Check sheet for the modelled part. Datum: model origin and axes. Units: mm. Face numbers are marked on the shaded views. Round coordinates to 2 decimals unless told otherwise and drop trailing zeros. Order: outer loops, then holes, each group sorted by start corner. A loop starts at its lowest first (then second) coordinate and runs counter-clockwise, first axis right, second up. Notation, with made-up numbers: M -7,-12.5 L 36,-12.5 A16 ccw 36,4.5 Z; hole C 28,73.5 d1. An arc over 180 degrees is marked long. One line per item, written item: value. Start each with the question number.
(1) Cross-section at B-B, the plane x = 65. Enter the section's corners in (y, z), and give its area (3 significant figures).
(2) Depth check by flat-ended pin: pin 1 Ø23.5 at (x, y) = (-6.5, 0) entering from +Z; pin 2 Ø4.5 at (y, z) = (-13.5, 4) entering from +X; pin 3 Ø2 at (x, z) = (-23, 6) entering from -Y. Enter the tip coordinate at first touch or a pass-through.
(3) Cross-section at A-A, the plane x = 15.5. Enter the section's corners in (y, z).
(4) Thickness scan on L1, parallel to X at y = -8, z = 3.75; L2, parallel to Z at x = 9, y = -16.5. Record the ranges inside material, lowest first.
(5) Release check for a two-part mould opening along X. For the marked faces 1 and 2 record: released by +X, released by -X, zero draft, split by the parting line, or undercut.
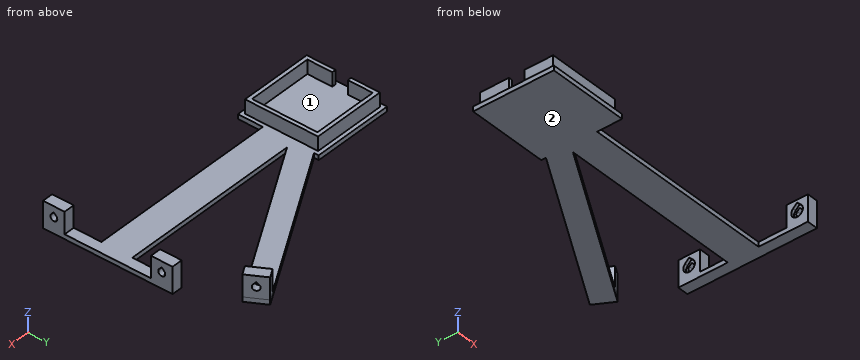
from build123d import *

# Parameters (mm, degrees)
F1_DEPTH  = 9
F2_W      = 123.8
F2_H      = 10
F3_DEPTH  = 3
F5_DEPTH  = 5
F6_W      = 14
F6_H      = 14
F7_DEPTH  = 2
F10_DEPTH = 2
F11_W     = 14
F11_H     = 14
F12_DEPTH = 5


with BuildPart() as f1:
    # F0 (on Top) → F1 (new body)
    with BuildSketch(Plane.XY):
        Polygon((-21.2, 21.2), (21.2, 21.2), (21.2, 0), (23.7, 0), (23.7, 23.7), (-23.7, 23.7), (-23.7, 5), (-21.2, 5), align=None)
        Polygon((23.7, 0), (21.2, 0), (21.2, -21.2), (-21.2, -21.2), (-21.2, -5), (-23.7, -5), (-23.7, -23.7), (23.7, -23.7), align=None)
    extrude(amount=F1_DEPTH)

    # F2 (on Top) → F3 (join)
    with BuildSketch(Plane.XY):
        Polygon((-26.2, 26.2), (-26.2, -26.2), (26.2, -26.2), (26.2, -10), (26.2, 0), (0, 0), (26.2, 15.1265770528), (26.2, 23.2094808214), (26.2, 26.2), align=None)
        Polygon((150, 40.1923788647), (150, 10), (157, 10), (157, 35), (157, 42), (150, 42), align=None)
        Polygon((26.2, 10), (26.2, 0), (150, 0), (150, 10), (31.3205080757, 10), align=None)
        Polygon((150, 0), (150, -10), (157, -10), (157, 10), (150, 10), align=None)
        Polygon((157, -10), (150, -10), (150, -40.1923788647), (150, -42), (157, -42), (157, -35), align=None)
        with Locations((88.1, -5)):
            Rectangle(F2_W, F2_H)
        Polygon((0, 0), (26.2, 0), (26.2, 10), (26.2, 15.1265770528), align=None)
        Polygon((126.4038105677, 81.0621778265), (26.2, 23.2094808214), (26.2, 15.1265770528), (129.9038105677, 75), align=None)
        Polygon((26.2, 15.1265770528), (26.2, 10), (31.3205080757, 10), (133.4038105677, 68.9378221735), (129.9038105677, 75), align=None)
        Polygon((132.4659883942, 84.5621778265), (126.4038105677, 81.0621778265), (129.9038105677, 75), (133.4038105677, 68.9378221735), (139.4659883942, 72.4378221735), align=None)
    extrude(amount=-F3_DEPTH)

    # F4 (on face) → F5 (join)
    with BuildSketch(Plane.YZ.offset(157)):
        Polygon((28, 0), (35, 0), (42, 0), (42, 14), (28, 14), align=None)
        with BuildLine():
            ThreePointArc((37.25, 7), (36.5909902577, 5.4090097423), (35, 4.75))
            ThreePointArc((35, 4.75), (33.4090097423, 5.4090097423), (32.75, 7))
            ThreePointArc((32.75, 7), (32.9212710518, 7.8610377228), (33.4090097423, 8.5909902577))
            Line((33.4090097423, 8.5909902577), (35, 10.1819805153))
            Line((35, 10.1819805153), (36.5909902577, 8.5909902577))
            ThreePointArc((36.5909902577, 8.5909902577), (37.0787289482, 7.8610377228), (37.25, 7))
        make_face(mode=Mode.SUBTRACT)
        Polygon((-35, 0), (-28, 0), (-28, 14), (-42, 14), (-42, 0), align=None)
        with BuildLine():
            ThreePointArc((-32.75, 7), (-33.4090097423, 5.4090097423), (-35, 4.75))
            ThreePointArc((-35, 4.75), (-36.5909902577, 5.4090097423), (-37.25, 7))
            ThreePointArc((-37.25, 7), (-37.0787289482, 7.8610377228), (-36.5909902577, 8.5909902577))
            Line((-36.5909902577, 8.5909902577), (-35, 10.1819805153))
            Line((-35, 10.1819805153), (-33.4090097423, 8.5909902577))
            ThreePointArc((-33.4090097423, 8.5909902577), (-32.9212710518, 7.8610377228), (-32.75, 7))
        make_face(mode=Mode.SUBTRACT)
    extrude(amount=-F5_DEPTH)

    # F6 (on face) → F7 (join)
    with BuildSketch(Plane(origin=(152, 0, 0), x_dir=(0, -1, 0), z_dir=(-1, 0, 0))):
        with Locations((-35, 7)):
            Rectangle(F6_W, F6_H)
        with BuildLine():
            ThreePointArc((-32.3483495706, 9.6516504294), (-31.5354517531, 8.4350628714), (-31.25, 7))
            ThreePointArc((-31.25, 7), (-35, 3.25), (-38.75, 7))
            ThreePointArc((-38.75, 7), (-38.4645482469, 8.4350628714), (-37.6516504294, 9.6516504294))
            Line((-37.6516504294, 9.6516504294), (-35, 12.3033008589))
            Line((-35, 12.3033008589), (-32.3483495706, 9.6516504294))
        make_face(mode=Mode.SUBTRACT)
        with Locations((35, 7)):
            Rectangle(F6_W, F6_H)
        with BuildLine():
            ThreePointArc((37.6516504294, 9.6516504294), (38.4645482469, 8.4350628714), (38.75, 7))
            ThreePointArc((38.75, 7), (35, 3.25), (31.25, 7))
            ThreePointArc((31.25, 7), (31.5354517531, 8.4350628714), (32.3483495706, 9.6516504294))
            Line((32.3483495706, 9.6516504294), (35, 12.3033008589))
            Line((35, 12.3033008589), (37.6516504294, 9.6516504294))
        make_face(mode=Mode.SUBTRACT)
    extrude(amount=F7_DEPTH)

    # F9 (on line) → F10 (join)
    with BuildSketch(Plane(origin=(129.9038105677, 75, 0), x_dir=(0.5, -0.8660254038, 0), z_dir=(-0.8660254038, -0.5, 0))):
        Polygon((-7, 0), (0, 0), (7, 0), (7, 14), (-7, 14), align=None)
        with BuildLine():
            ThreePointArc((3.75, 7), (2.6516504294, 4.3483495706), (0, 3.25))
            ThreePointArc((0, 3.25), (-3.4645482469, 5.5649371286), (-2.6516504294, 9.6516504294))
            Line((-2.6516504294, 9.6516504294), (0, 12.3033008589))
            Line((0, 12.3033008589), (2.6516504294, 9.6516504294))
            ThreePointArc((2.6516504294, 9.6516504294), (3.4645482469, 8.4350628714), (3.75, 7))
        make_face(mode=Mode.SUBTRACT)
    extrude(amount=-F10_DEPTH)

    # F11 (on face) → F12 (join)
    with BuildSketch(Plane(origin=(131.6358613752, 76, 0), x_dir=(-0.5, 0.8660254038, 0), z_dir=(0.8660254038, 0.5, 0))):
        with Locations((0, 7)):
            Rectangle(F11_W, F11_H)
        with BuildLine():
            Line((-2.6516504294, 9.6516504294), (0, 12.3033008589))
            Line((0, 12.3033008589), (2.6516504294, 9.6516504294))
            ThreePointArc((2.6516504294, 9.6516504294), (0, 3.25), (-2.6516504294, 9.6516504294))
        make_face(mode=Mode.SUBTRACT)
        with BuildLine():
            Line((2.6516504294, 9.6516504294), (0, 12.3033008589))
            Line((0, 12.3033008589), (-2.6516504294, 9.6516504294))
            ThreePointArc((-2.6516504294, 9.6516504294), (0, 3.25), (2.6516504294, 9.6516504294))
        make_face()
        with BuildLine():
            ThreePointArc((1.5909902577, 8.5909902577), (2.0787289482, 7.8610377228), (2.25, 7))
            ThreePointArc((2.25, 7), (0, 4.75), (-2.25, 7))
            ThreePointArc((-2.25, 7), (-2.0787289482, 7.8610377228), (-1.5909902577, 8.5909902577))
            Line((-1.5909902577, 8.5909902577), (0, 10.1819805153))
            Line((0, 10.1819805153), (1.5909902577, 8.5909902577))
        make_face(mode=Mode.SUBTRACT)
    extrude(amount=F12_DEPTH)


solid = f1.part
Values found:
1. outline: M -10,-3 L 10,-3 L 10,0 L -10,0 Z; M 29.44,-3 L 45.61,-3 L 45.61,0 L 29.44,0 Z
1. area: 108 mm^2
2. pin 1: z = 0
2. pin 2: x = 23.7
2. pin 3: y = -23.7
3. outline: M -26.2,-3 L 26.2,-3 L 26.2,0 L 23.7,0 L 23.7,9 L 21.2,9 L 21.2,0 L -21.2,0 L -21.2,9 L -23.7,9 L -23.7,0 L -26.2,0 Z
4. L1: -23.7 to -21.2, 21.2 to 23.7
4. L2: -3 to 0
5. face 1: undercut
5. face 2: zero draft
